Here's how the part is built. I have some questions about the finished solid (model axes, mm). Give positions to 0.01 mm unless a question says otherwise; leave off trailing zeros. Loops run counter-clockwise (first coordinate to the right, second up) from the corner with the lowest first, then second, coordinate; pieces in that order, holes last.
Q1. I'm going to push flat-ended pins straight in: P1, Ø1.5, axis at x = 47.5, z = 4, coming from the -Y side; P2, Ø7.5, axis at x = 57.15, y = 12.7, coming from the +Z side. Where does each tip first touch, or does it pass through?
Q2. Suppose I cut it at B-B (x = 12.7). List the corners of the cut face in (y, z) for me, and give its area (3 significant figures).
Q3. Suppose I cut it at A-A (y = 38.1). List the corners of the cut face in (x, z) for me, and give its area (3 significant figures).
Q4. I need wall thicknesses on probe 1 along Y at (x, z) = (12.7, 3.7); probe 2 along Y at (x, z) = (40, 2.95); probe 3 along Y at (x, z) = (38.1, 1.9). Which ranges of each line are inside material? Lowest first, please.
Q5. Thinking about a two-plate mould opening in Y: for faces 1 (the face through (38, 39, 0)), 2 (the face through (39, 76.2, 2)), 3 (the face through (38, 0, 2)), 4 (the face through (64.6, 61.39, 2.41)), which applies, pulls with the +Y half, pulls with the -Y half, needs draft (parallel to the pull), parting line crosses it, or undercut?
Q6. Suppose I cut it at C-C (z = 3.1). List the corners of the cut face in (x, y) for me.
Q7. Suppose I cut it at D-D (x = 57.15). List the corners of the cut face in (y, z) for me, and give its area (3 significant figures).
Autodesk Inventor part; units mm, degrees
ref_plane "YZ Plane" through (0, 0, 0) normal (1, 0, 0) x (0, 1, 0)
ref_plane "XZ Plane" through (0, 0, 0) normal (0, 1, 0) x (-1, 0, 0)
ref_plane "XY Plane" through (0, 0, 0) normal (0, 0, 1) x (1, 0, 0)
sketch "Sketch1" plane through (0, 0, 0) normal (0, 0, 1) x (1, 0, 0)
  line L0 (0, 0) -> (76.2, 0)
  line L1 (76.2, 0) -> (76.2, 76.2)
  line L2 (76.2, 76.2) -> (0, 76.2)
  line L3 (0, 76.2) -> (0, 0)
  dimension "d0" = 76.2
  dimension "d1" = 76.2
extrude "Extrusion1" add sketch "Sketch1" along normal blind 4.7625
sketch "Sketch2" plane through (0, 0, 4.7625) normal (0, 0, 1) x (1, 0, 0)
  line L0 (0, 0) -> (0, 76.2)
  line L1 (76.2, 0) -> (0, 0)
  circle A0 centre (57.15, 12.7) radius 6.35
  dimension "d4" = 12.7
  dimension "d5" = 12.7
  dimension "d6" = 57.15
extrude "Extrusion2" cut sketch "Sketch2" against normal up to next
sketch "Sketch3" plane through (0, 0, 4.7625) normal (0, 0, 1) x (1, 0, 0)
  line L0 (0, 0) -> (0, 76.2)
  line L1 (0, 76.2) -> (76.2, 76.2)
  circle A0 centre (12.7, 63.5) radius 2.3813
  dimension "d9" = 4.7625
  dimension "d10" = 12.7
  dimension "d11" = 12.7
extrude "Extrusion3" cut sketch "Sketch3" against normal up to next
pattern_linear "Rectangular Pattern1" count 3 spacing 25.4 along (1, 0, 0) of "Extrusion3"
pattern_linear "Rectangular Pattern2" count 3 spacing 25.4 along (0, -1, 0) of "Extrusion3"
properties part number "Frame_TopRearRollerPlate"
Solutions:
1. P1: stops at y = 0
1. P2: passes through
2. outline: (0, 0) - (10.32, 0) - (10.32, 4.76) - (0, 4.76) - close; (15.08, 0) - (35.72, 0) - (35.72, 4.76) - (15.08, 4.76) - close; (40.48, 0) - (61.12, 0) - (61.12, 4.76) - (40.48, 4.76) - close; (65.88, 0) - (76.2, 0) - (76.2, 4.76) - (65.88, 4.76) - close
2. area: 295 mm2
3. outline: (0, 0) - (10.32, 0) - (10.32, 4.76) - (0, 4.76) - close; (15.08, 0) - (76.2, 0) - (76.2, 4.76) - (15.08, 4.76) - close
3. area: 340 mm2
4. probe 1: y = 0 to 10.32, 15.08 to 35.72, 40.48 to 61.12, 65.88 to 76.2
4. probe 2: y = 0 to 62.06, 64.94 to 76.2
4. probe 3: y = 0 to 61.12, 65.88 to 76.2
5. face 1: needs draft
5. face 2: pulls with the +Y half
5. face 3: pulls with the -Y half
5. face 4: undercut
6. outline: (0, 0) - (76.2, 0) - (76.2, 76.2) - (0, 76.2) - close; hole circle Ø4.76 at (12.7, 12.7); hole circle Ø4.76 at (12.7, 38.1); hole circle Ø4.76 at (12.7, 63.5); hole circle Ø4.76 at (38.1, 63.5); hole circle Ø12.7 at (57.15, 12.7); hole circle Ø4.76 at (63.5, 63.5)
7. outline: (0, 0) - (6.35, 0) - (6.35, 4.76) - (0, 4.76) - close; (19.05, 0) - (76.2, 0) - (76.2, 4.76) - (19.05, 4.76) - close
7. area: 302 mm2
